The listing builds one solid part. Answer for the finished solid, in the listing's coordinates (mm). A direction names the side the tool comes from. Coordinates: 2 decimals unless noted, no trailing zeros. Order: outer loops, then holes, each group sorted by start corner. A loop starts at its lowest first (then second) coordinate and runs counter-clockwise, first axis right, second up. Notation, with made-up numbers: (41, 68.25) -> (45, 68.25) arc R33 ccw to (45, 98.25) -> close; hole circle Ø9 at (-20, -33). An arc over 180 degrees is marked (long way). Write item = value, one per line. Start each with the question number.
```python
from build123d import *

# Parameters (mm, degrees)
CHAMFER1_SIZE           = 3
CHAMFER2_SIZE           = 2
SKETCH2_R               = 3
CUT_EXTRUDE1_DEPTH      = 17
CUT_EXTRUDE1_DEPTH_BACK = 17


with BuildPart() as part:
    # Sketch1 → Revolve1 (revolve)
    with BuildSketch(Plane.XY):
        Polygon((155, 0), (155, 16), (135, 16), (135, 9), (82, 9), (82, 7), (80, 7), (80, 9), (60, 9), (60, 7), (58, 7), (58, 9), (0, 9), (0, 0), align=None)
    revolve(axis=Axis((0, 0, 0), (1, 0, 0)))

    # Chamfer1
    chamfer1_edges = [part.edges().sort_by_distance(p)[0] for p in [
        (135, -16, 0),
        (155, -16, 0),
    ]]
    chamfer(chamfer1_edges, length=CHAMFER1_SIZE)

    # Chamfer2
    chamfer2_edges = [part.edges().sort_by_distance(p)[0] for p in [
        (0, -9, 0),
    ]]
    chamfer(chamfer2_edges, length=CHAMFER2_SIZE)

    # Sketch2 → Cut-Extrude1 (cut, two sides)
    with BuildSketch(Plane.XY) as cut_extrude1_sk:
        with Locations((145, 0)):
            Circle(SKETCH2_R)
    extrude(amount=CUT_EXTRUDE1_DEPTH, mode=Mode.SUBTRACT)
    extrude(cut_extrude1_sk.sketch, amount=-CUT_EXTRUDE1_DEPTH_BACK, mode=Mode.SUBTRACT)


solid = part.part
```
Item 1: For a pull along X with two mould halves and no side action, classify faces 1 (the cylindrical face through (29.608, -1.172, 8.923)), 2 (the cylindrical face through (80.986, 6.466, -2.681)), 3 (the flat face through (135, 3, 9)), 4 (the conical face through (154.81, 12.58, 3.96)) as pulls with the +X half, pulls with the -X half, needs draft (parallel to the pull), parting line crosses it, or undercut.
Item 2: Consider probe 1 along X at (y, z) = (0, 10.5); probe 2 along Z at (x, y) = (108, -0.5); probe 3 along X at (y, z) = (-2.5, 14). Determine where each line is inside the solid, lowest interval first.
Item 3: Section A-A, the plane x = 41 is taken. Give the vertices of the cut face in (y, z).
Item 4: Which of the six approach directions +Z, -Z, +X, -X, +Y, -Y give full straight-line access (tool end or side, diameter ignored) to faces 5 (the flat face through (58, 0, -7.3)), 6 (the cylindrical face through (69.86, -1.172, 8.923)), 7 (the flat face through (155, 0, 0))?
Item 5: Section B-B, the plane x = 145 is taken. Give the vertices of the cut face in (y, z).
Item 6: Each of these flat-tipped pins is pushed along its axis until it touches: pin 1 (14.5 mm diameter, centred on y = -2, z = -4, fed in from -X); pin 2 (1.5 mm diameter, centred on y = -10, z = -11.5, fed in from -X); pin 3 (5 mm diameter, centred on x = 63.5, y = -9.5, fed in from +Z); pin 4 (8 mm diameter, centred on x = 99.5, y = -1, fed in from +Z). Where does it stop, or does it pass through?
A:
q1.face_1 = needs draft
q1.face_2 = undercut
q1.face_3 = pulls with the -X half
q1.face_4 = pulls with the +X half
q2.probe_1 = 135 to 142, 148 to 155
q2.probe_2 = -8.99 to 8.99
q2.probe_3 = 136.22 to 143.34, 146.66 to 153.78
q3.outline = circle Ø18 at (0, 0)
q4.face_5 = none
q4.face_6 = -X
q4.face_7 = +Z, -Z, +X, +Y, -Y
q5.outline = (-3, -15.72) -> (-3, 15.72) arc R16 ccw to start; (3, -15.72) arc R16 ccw to (3, 15.72) -> close
q6.pin_1 = 0
q6.pin_2 = 136.49
q6.pin_3 = 5.66
q6.pin_4 = 9
